Geometry: final body of the model. Coordinates: model frame, mm. Face numbers are marked on the shaded views. A direction names the side the tool comes from. Coordinates: 2 decimals unless noted, no trailing zeros. Order: outer loops, then holes, each group sorted by start corner. A loop starts at its lowest first (then second) coordinate and runs counter-clockwise, first axis right, second up. Notation, with made-up numbers: (51.25, 39.5) - (105.25, 39.5) arc R28 cw to (105.25, 70.5) - close; hole circle Ø8 at (-15, -13.5). An arc over 180 degrees is marked (long way). Use a Markdown table: item, result. Add a question column.
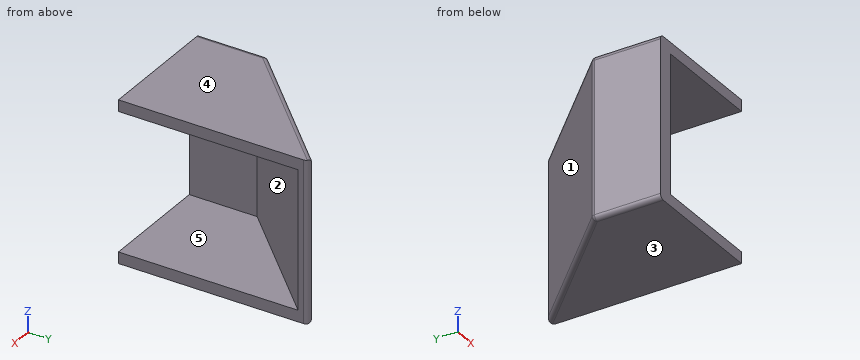
```python
from build123d import *

# Parameters (mm, degrees)
BOSS_EXTRUDE1_DEPTH              = 22.606
CUT_EXTRUDE1_REACH               = 21.561
CUT_EXTRUDE1_OFFSET_FROM_SURFACE = 1.6
SKETCH2_W                        = 19.406
SKETCH2_H                        = 16.360512242
BOSS_EXTRUDE2_DEPTH              = 9.525
FILLET1_R                        = 0.635


with BuildPart() as part:
    # Sketch1 → Boss-Extrude1 (new body)
    with BuildSketch(Plane.XY):
        Polygon((0, 0), (17.960512242, 17.960512242), (17.960512242, 0), align=None)
    extrude(amount=BOSS_EXTRUDE1_DEPTH)

    # Cut-Extrude1: up to this face of the body (flat: up to its plane, moved by the offset)
    cut_extrude1_end = Plane(part.part.faces().sort_by_distance((8.980256121, 8.980256121, 11.303))[0]).offset(-CUT_EXTRUDE1_OFFSET_FROM_SURFACE)
    # Sketch2 → Cut-Extrude1 (cut, up to the picked face)
    with BuildSketch(Plane(origin=(17.960512242, 0, 0), x_dir=(0, 0, -1), z_dir=(1, 0, 0)), mode=Mode.PRIVATE) as cut_extrude1_sk1:
        with Locations((-11.303, 8.180256121)):
            Rectangle(SKETCH2_W, SKETCH2_H)
    cut_extrude1_tool1 = split(extrude(cut_extrude1_sk1.sketch, amount=-CUT_EXTRUDE1_REACH, mode=Mode.PRIVATE), bisect_by=cut_extrude1_end, keep=Keep.BOTH, mode=Mode.PRIVATE)
    add(cut_extrude1_tool1.solids().sort_by_distance((17.960512, 8.180256, 11.303))[0], mode=Mode.SUBTRACT)

    # Sketch3 → Boss-Extrude2 (add)
    with BuildSketch(Plane.XZ):
        Polygon((17.960512242, 22.606), (0, 22.606), (0, 0), (17.960512242, 0), (17.960512242, 1.6), (2.2627417, 1.6), (2.2627417, 21.006), (17.960512242, 21.006), align=None)
    extrude(amount=BOSS_EXTRUDE2_DEPTH)

    # Fillet1
    fillet1_edges = [part.edges().sort_by_distance(p)[0] for p in [
        (8.980256121, 8.980256121, 22.606),
        (0, -4.7625, 22.606),
        (0, -4.7625, 0),
        (8.980256121, 8.980256121, 0),
        (0, 0, 11.303),
        (17.960512242, 17.960512242, 11.303),
    ]]
    fillet(fillet1_edges, radius=FILLET1_R)


solid = part.part
```
1) Ray query, line 1 along Z through (x, y) = (6.5, 1.5); line 2 along X through (y, z) = (-3.5, 12.75); line 3 along Z through (x, y) = (13.5, 12.75). Return the intervals inside material, ascending.
2) Section A-A (z = 6). Return loops of the section in (x, y) (1 decimal), then the cut area to 3 significant figures.
3) Set-up query: the marked faces 4 and 5. Return all of +Z, -Z, +X, -X, +Y, -Y with unobstructed straight access to the full face (end or side cutting, diameter ignored); none if empty.
4) Pin query (flat end, axial travel): pin 1 (6 mm diameter, centred on y = 5.5, z = 18, fed in from -X); pin 2 (4 mm diameter, centred on y = -0.5, z = 14, fed in from +X); pin 3 (2 mm diameter, centred on y = 13.5, z = 19, fed in from +X). Return the tip coordinate at first contact, or that it passes through.
5) Draft query along Z for the marked faces 1, 2 and 3. Return one class per face: pulls with the +Z half, pulls with the -Z half, needs draft (parallel to the pull), parting line crosses it, or undercut.
6) Section B-B (y = -2.5). Return loops of the section in (x, z) (3 decimals), then the cut area to 3 significant figures.
Values follow:
| question | item | result |
|---|---|---|
| 1 | line 1 | z = 0 to 1.6, 21.01 to 22.61 |
| 1 | line 2 | x = 0 to 2.26 |
| 1 | line 3 | z = 0.01 to 22.6 |
| 2 | outline | (0, -9.5) - (2.3, -9.5) - (2.3, 0) - (18, 15.7) - (18, 16.4) arc R0.6 ccw to (16.9, 16.9) - (0.2, 0.2) arc R0.6 ccw to (0, -0.3) - close |
| 2 | area | 59.1 mm² |
| 3 | face 4 | +Z, +X, -X, +Y, -Y |
| 3 | face 5 | +X, -Y |
| 4 | pin 1 | stops at x = 2.5 |
| 4 | pin 2 | stops at x = 3.76 |
| 4 | pin 3 | stops at x = 16.76 |
| 5 | face 1 | needs draft |
| 5 | face 2 | undercut |
| 5 | face 3 | pulls with the -Z half |
| 6 | outline | (0, 0.635) arc R0.635 ccw to (0.635, 0) - (17.961, 0) - (17.961, 1.6) - (2.263, 1.6) - (2.263, 21.006) - (17.961, 21.006) - (17.961, 22.606) - (0.635, 22.606) arc R0.635 ccw to (0, 21.971) - close |
| 6 | area | 101 mm² |
